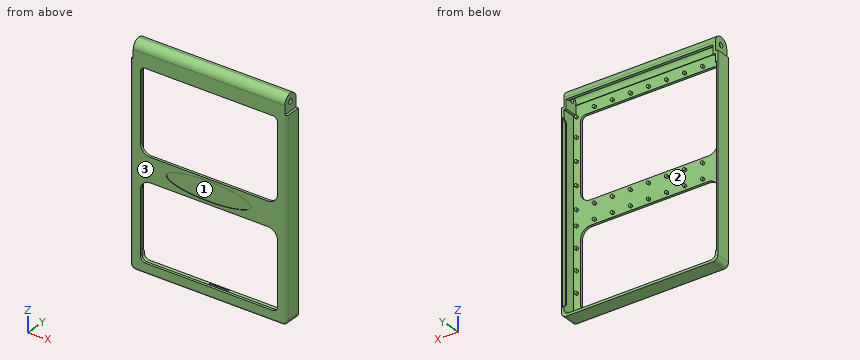
from build123d import *

# Parameters (mm, degrees)
SALIENTE_EXTRUIR1_DEPTH     = 13
CORTAR_EXTRUIR7_DEPTH       = 11
CORTAR_EXTRUIR9_DEPTH       = 140
CROQUIS10_R                 = 4.5
CORTAR_EXTRUIR10_DEPTH      = 122
CROQUIS11_W                 = 122
CROQUIS11_H                 = 12.524990812
CORTAR_EXTRUIR12_DEPTH      = 11
CORTAR_EXTRUIR13_DEPTH      = 130
CORTAR_EXTRUIR13_DEPTH_BACK = 130
CROQUIS12_R                 = 2
REDONDEO1_R                 = 1
CORTAR_EXTRUIR14_DEPTH      = 1
CORTAR_EXTRUIR15_DEPTH      = 1
CORTAR_EXTRUIR17_DEPTH      = 4
CROQUIS21_RX                = 35
CROQUIS21_RY                = 8
CORTAR_EXTRUIR19_DEPTH      = 0.4
CROQUIS22_R                 = 1.2
SALIENTE_EXTRUIR3_DEPTH     = 1.8
CROQUIS25_R                 = 0.7
CORTAR_EXTRUIR20_DEPTH      = 16


with BuildPart() as part:
    # Croquis1 → Saliente-Extruir1 (new body)
    with BuildSketch(Plane(origin=(0, 0, 0), x_dir=(1, 0, 0), z_dir=(0, 1, 0))):
        with BuildLine():
            Line((130, 0), (128, 0))
            Line((128, 0), (128, -14))
            Line((128, -14), (2, -14))
            Line((2, -14), (2, 0))
            Line((2, 0), (0, 0))
            Line((0, 0), (0, 160))
            ThreePointArc((0, 160), (1.171572875, 162.828427125), (4, 164))
            Line((4, 164), (126, 164))
            ThreePointArc((126, 164), (128.828427125, 162.828427125), (130, 160))
            Line((130, 160), (130, 0))
        make_face()
    extrude(amount=SALIENTE_EXTRUIR1_DEPTH)

    # Croquis7 → Cortar-Extruir7 (cut)
    with BuildSketch(Plane(origin=(0, 13, 0), x_dir=(1, 0, 0), z_dir=(0, 1, 0))):
        with BuildLine():
            ThreePointArc((124, 162), (126.828427125, 160.828427125), (128, 158))
            Line((128, 158), (128, 2))
            Line((128, 2), (2, 2))
            Line((2, 2), (2, 158))
            ThreePointArc((2, 158), (3.171572875, 160.828427125), (6, 162))
            Line((6, 162), (62.001239157, 162))
            Line((62.001239157, 162), (124, 162))
        make_face()
    extrude(amount=-CORTAR_EXTRUIR7_DEPTH, mode=Mode.SUBTRACT)

    # Croquis8 → Cortar-Extruir9 (cut)
    with BuildSketch(Plane(origin=(128, 0, 0), x_dir=(0, 0, -1), z_dir=(1, 0, 0))):
        with BuildLine():
            ThreePointArc((-14, 6.5), (-12.096194078, 11.096194078), (-7.5, 13))
            Line((-7.5, 13), (-14, 13))
            Line((-14, 13), (-14, 6.5))
        make_face()
        with BuildLine():
            Line((-14, 0), (-7.5, 0))
            ThreePointArc((-7.5, 0), (-12.096194078, 1.903805922), (-14, 6.5))
            Line((-14, 6.5), (-14, 0))
        make_face()
    extrude(amount=-CORTAR_EXTRUIR9_DEPTH, mode=Mode.SUBTRACT)

    # Croquis10 → Cortar-Extruir10 (cut)
    with BuildSketch(Plane(origin=(4, 0, 0), x_dir=(0, 0, -1), z_dir=(1, 0, 0))):
        with Locations(Location((-7.5, 6.5, 0), (0, 0, 180))):
            Circle(CROQUIS10_R)
    extrude(amount=CORTAR_EXTRUIR10_DEPTH, mode=Mode.SUBTRACT)

    # Croquis11 → Cortar-Extruir12 (cut)
    with BuildSketch(Plane(origin=(0, 13, 0), x_dir=(1, 0, 0), z_dir=(0, 1, 0))):
        Polygon((4, 2), (4, -5.5), (6, -5.5), (126, -5.5), (126, 2), align=None)
        with Locations((65, 8.262495406)):
            Rectangle(CROQUIS11_W, CROQUIS11_H)
    extrude(amount=-CORTAR_EXTRUIR12_DEPTH, mode=Mode.SUBTRACT)

    # Croquis12 → Cortar-Extruir13 (cut, two sides: drawn at the far end of the back side and taken through both)
    with BuildSketch(Plane(origin=(4, 0, 0), x_dir=(0, 0, -1), z_dir=(1, 0, 0)).offset(-CORTAR_EXTRUIR13_DEPTH_BACK)):
        with Locations((-7.5, 6.5)):
            Circle(CROQUIS12_R)
    extrude(amount=CORTAR_EXTRUIR13_DEPTH + CORTAR_EXTRUIR13_DEPTH_BACK, mode=Mode.SUBTRACT)

    # Redondeo1
    redondeo1_edges = [part.edges().sort_by_distance(p)[0] for p in [
        (128.828427125, 0, -162.828427125),
        (130, 0, -80),
        (0, 0, -80),
        (1.171572875, 0, -162.828427125),
        (65, 0, -164),
    ]]
    fillet(redondeo1_edges, radius=REDONDEO1_R)

    # Croquis17 → Cortar-Extruir14 (cut)
    with BuildSketch(Plane(origin=(2, 0, 0), x_dir=(0, 0, -1), z_dir=(1, 0, 0))):
        Polygon((153, 10), (11, 10), (8, 13), (156, 13), align=None)
    extrude(amount=-CORTAR_EXTRUIR14_DEPTH, mode=Mode.SUBTRACT)

    # Croquis19 → Cortar-Extruir15 (cut)
    with BuildSketch(Plane(origin=(128, 0, 0), x_dir=(0, 0, -1), z_dir=(1, 0, 0))):
        Polygon((11, 10), (153, 10), (156, 13), (8, 13), align=None)
    extrude(amount=CORTAR_EXTRUIR15_DEPTH, mode=Mode.SUBTRACT)

    # Croquis20 → Cortar-Extruir17 (cut)
    with BuildSketch(Plane.XZ):
        with BuildLine():
            Line((85, -72), (114, -72))
            ThreePointArc((114, -72), (119.656854249, -69.656854249), (122, -64))
            Line((122, -64), (122, -24.159979327))
            Line((122, -24.159979327), (122, -8))
            ThreePointArc((122, -8), (120.828427125, -5.171572875), (118, -4))
            Line((118, -4), (12, -4))
            ThreePointArc((12, -4), (9.171572875, -5.171572875), (8, -8))
            Line((8, -8), (8, -64))
            ThreePointArc((8, -64), (10.343145751, -69.656854249), (16, -72))
            Line((16, -72), (45, -72))
            Line((45, -72), (85, -72))
        make_face()
        with BuildLine():
            Line((45, -92), (85, -92))
            Line((85, -92), (114, -92))
            ThreePointArc((114, -92), (119.656854249, -94.343145751), (122, -100))
            Line((122, -100), (122, -152))
            ThreePointArc((122, -152), (120.828427125, -154.828427125), (118, -156))
            Line((118, -156), (68.281659804, -156))
            Line((68.281659804, -156), (12, -156))
            ThreePointArc((12, -156), (9.171572875, -154.828427125), (8, -152))
            Line((8, -152), (8, -100))
            ThreePointArc((8, -100), (10.343145751, -94.343145751), (16, -92))
            Line((16, -92), (45, -92))
        make_face()
    extrude(amount=-CORTAR_EXTRUIR17_DEPTH, mode=Mode.SUBTRACT)

    # Croquis21 → Cortar-Extruir19 (cut)
    with BuildSketch(Plane.XZ):
        with Locations(Location((64.555474057, -81.656567249), (0, 0, 180))):
            Ellipse(CROQUIS21_RX, CROQUIS21_RY)
    extrude(amount=-CORTAR_EXTRUIR19_DEPTH, mode=Mode.SUBTRACT)

    # Croquis22 → Saliente-Extruir3 (add)
    with BuildSketch(Plane(origin=(0, 2, 0), x_dir=(1, 0, 0), z_dir=(0, 1, 0))):
        with Locations(Location((20, 159, 0), (0, 0, 270))):
            Circle(CROQUIS22_R)
        with Locations(Location((35, 159, 0), (0, 0, 270))):
            Circle(CROQUIS22_R)
        with Locations(Location((50, 159, 0), (0, 0, 270))):
            Circle(CROQUIS22_R)
        with Locations(Location((65, 159, 0), (0, 0, 270))):
            Circle(CROQUIS22_R)
        with Locations(Location((80, 159, 0), (0, 0, 270))):
            Circle(CROQUIS22_R)
        with Locations(Location((95, 159, 0), (0, 0, 270))):
            Circle(CROQUIS22_R)
        with Locations(Location((110, 159, 0), (0, 0, 270))):
            Circle(CROQUIS22_R)
        with Locations(Location((125, 159, 0), (0, 0, 270))):
            Circle(CROQUIS22_R)
        with Locations(Location((5, 159, 0), (0, 0, 270))):
            Circle(CROQUIS22_R)
        with Locations(Location((5, 89, 0), (0, 0, 270))):
            Circle(CROQUIS22_R)
        with Locations(Location((20, 89, 0), (0, 0, 270))):
            Circle(CROQUIS22_R)
        with Locations(Location((35, 89, 0), (0, 0, 270))):
            Circle(CROQUIS22_R)
        with Locations(Location((50, 89, 0), (0, 0, 270))):
            Circle(CROQUIS22_R)
        with Locations(Location((65, 89, 0), (0, 0, 270))):
            Circle(CROQUIS22_R)
        with Locations(Location((80, 89, 0), (0, 0, 270))):
            Circle(CROQUIS22_R)
        with Locations(Location((95, 89, 0), (0, 0, 270))):
            Circle(CROQUIS22_R)
        with Locations(Location((110, 89, 0), (0, 0, 270))):
            Circle(CROQUIS22_R)
        with Locations(Location((125, 89, 0), (0, 0, 270))):
            Circle(CROQUIS22_R)
        with Locations(Location((125, 76.396213734, 0), (0, 0, 270))):
            Circle(CROQUIS22_R)
        with Locations(Location((110, 76.396213734, 0), (0, 0, 270))):
            Circle(CROQUIS22_R)
        with Locations(Location((80, 76.396213734, 0), (0, 0, 270))):
            Circle(CROQUIS22_R)
        with Locations(Location((65, 76.396213734, 0), (0, 0, 270))):
            Circle(CROQUIS22_R)
        with Locations(Location((95, 76.396213734, 0), (0, 0, 270))):
            Circle(CROQUIS22_R)
        with Locations(Location((50, 76.396213734, 0), (0, 0, 270))):
            Circle(CROQUIS22_R)
        with Locations(Location((20, 76.396213734, 0), (0, 0, 270))):
            Circle(CROQUIS22_R)
        with Locations(Location((35, 76.396213734, 0), (0, 0, 270))):
            Circle(CROQUIS22_R)
        with Locations(Location((5, 76.396213734, 0), (0, 0, 270))):
            Circle(CROQUIS22_R)
        with Locations(Location((20, 1, 0), (0, 0, 270))):
            Circle(CROQUIS22_R)
        with Locations(Location((35, 1, 0), (0, 0, 270))):
            Circle(CROQUIS22_R)
        with Locations(Location((50, 1, 0), (0, 0, 270))):
            Circle(CROQUIS22_R)
        with Locations(Location((65, 1, 0), (0, 0, 270))):
            Circle(CROQUIS22_R)
        with Locations(Location((80, 1, 0), (0, 0, 270))):
            Circle(CROQUIS22_R)
        with Locations(Location((95, 1, 0), (0, 0, 270))):
            Circle(CROQUIS22_R)
        with Locations(Location((110, 1, 0), (0, 0, 270))):
            Circle(CROQUIS22_R)
        with Locations(Location((5, 38.698106867, 0), (0, 0, 270))):
            Circle(CROQUIS22_R)
        with Locations(Location((125, 38.698106867, 0), (0, 0, 270))):
            Circle(CROQUIS22_R)
        with Locations(Location((5, 57.5471603, 0), (0, 0, 270))):
            Circle(CROQUIS22_R)
        with Locations(Location((125, 57.5471603, 0), (0, 0, 270))):
            Circle(CROQUIS22_R)
        with Locations(Location((5, 19.849053433, 0), (0, 0, 270))):
            Circle(CROQUIS22_R)
        with Locations(Location((125, 19.849053433, 0), (0, 0, 270))):
            Circle(CROQUIS22_R)
        with Locations(Location((125, 4, 0), (0, 0, 270))):
            Circle(CROQUIS22_R)
        with Locations(Location((5, 4, 0), (0, 0, 270))):
            Circle(CROQUIS22_R)
        with Locations(Location((125, 141.5, 0), (0, 0, 270))):
            Circle(CROQUIS22_R)
        with Locations(Location((125, 124, 0), (0, 0, 270))):
            Circle(CROQUIS22_R)
        with Locations(Location((125, 106.5, 0), (0, 0, 270))):
            Circle(CROQUIS22_R)
        with Locations(Location((5, 141.5, 0), (0, 0, 270))):
            Circle(CROQUIS22_R)
        with Locations(Location((5, 124, 0), (0, 0, 270))):
            Circle(CROQUIS22_R)
        with Locations(Location((5, 106.5, 0), (0, 0, 270))):
            Circle(CROQUIS22_R)
    extrude(amount=SALIENTE_EXTRUIR3_DEPTH)

    # Croquis25 → Cortar-Extruir20 (cut)
    with BuildSketch(Plane(origin=(73, 0, 0), x_dir=(0, 0, -1), z_dir=(1, 0, 0))):
        with Locations((162, 11.2)):
            Circle(CROQUIS25_R)
    extrude(amount=-CORTAR_EXTRUIR20_DEPTH, mode=Mode.SUBTRACT)


solid = part.part
Work out the finished part from the listing and answer in its coordinate system (mm). Face numbers are marked on the shaded views. Round coordinates to 2 decimals unless told otherwise and drop trailing zeros. Put each result on its own line as item: value. Start each with the question number.
Q1. Straight lines are drawn through the part: L1, parallel to Z at x = 80, y = 1; L2, parallel to X at y = 7, z = -58; L3, parallel to Z at x = 61, y = 7. For each, find the intervals that lie inside material, in ascending order. Write a range as [from, to].
Q2. Section A-A, the plane x = 40.5 is taken. Give the number of separate pieces and of enclosed holes in the cut face, and give its area (3 significant figures).
Q3. For a pull along X with two mould halves and no side action, classify the marked faces 1, 2 and 3 as pulls with the +X half, pulls with the -X half, needs draft (parallel to the pull), parting line crosses it, or undercut.
Q4. Flat-ended cylindrical pins translate along their axes: pin 1 (1.2 mm diameter, centred on x = 5.5, z = -3.5, fed in from +Y); pin 2 (0.5 mm diameter, centred on x = 1.5, z = -106.5, fed in from +Y); pin 3 (6.5 mm diameter, centred on y = 8, z = 10, fed in from -X); pin 4 (1.6 mm diameter, centred on y = 0.5, z = -29, fed in from -X). Find the tip coordinate at first contact, or state that the pin passes through.
Findings below:
1. L1: z = [-164, -156], [-92, -72], [-4, 10.96]
1. L2: x = [0, 2], [128, 130]
1. L3: z = [-164, -162], [11.97, 13.98]
2. separate pieces: 3
2. enclosed holes: 0
2. area: 135 mm^2
3. face 1: undercut
3. face 2: undercut
3. face 3: needs draft
4. pin 1: stops at y = 3.8
4. pin 2: stops at y = 10
4. pin 3: stops at x = 2
4. pin 4: stops at x = 0
